Geometry: final body of the model. Coordinates: model frame, mm. Face numbers are marked on the shaded views. A direction names the side the tool comes from. Give positions to 0.01 mm unless a question says otherwise; leave off trailing zeros. Loops run counter-clockwise (first coordinate to the right, second up) from the corner with the lowest first, then second, coordinate; pieces in that order, holes last. Notation, with made-up numbers: (35, 64.25) -> (69, 64.25) arc R16 ccw to (69, 68.25) -> close; hole circle Ø11 at (-27.75, 89.5). An arc over 180 degrees is marked (long way). Answer in a Markdown table with one row per item. Add a question column.
1) Line query: line 1 (X direction, y = 60.5, z = 172); line 2 (X direction, y = 60, z = 145.5); line 3 (Z direction, x = -308.8, y = 196.5). Output: solid intervals per line, ascending. Write a range as from..to.
2) First-contact query: P1, Ø3.5, axis at x = -308.5, y = 141.5, coming from the +Z side; P2, Ø5.5, axis at y = 141, z = 176, coming from the -X side; P3, Ø3.5, axis at y = 207.5, z = 187.5, coming from the +X side. Flat tips, straight axial feed; report the tip coordinate or a pass-through.
3) Access query for the marked faces 1, 2 and 3. Directions: +Z, -Z, +X, -X, +Y, -Y. A direction counts if a zero-diameter tool reaches every point of the face in a straight line with its end or side. Return the directions, or none.
4) Draft query along X for the marked faces 4, 5 and 6. Return one class per face: +X half, -X half, draft (parallel to the pull), parting line (faces both ways), or undercut.
5) Section query C-C (x = -108). Return the cut outline in (y, z), plus the area to 3 significant figures.
6) Section query A-A (y = 176). Return the cut outline in (x, z), plus the area to 3 significant figures.
7) Section query B-B (z = 85.5). Return the cut outline in (x, y).
```python
from build123d import *

# Parameters (mm, degrees)
BASE_FLANGE1_DEPTH             = 186
EDGE_FLANGE1_DEPTH             = 613
M6_CLEARANCE_HOLE1_D           = 6.4
EDGE_FLANGE2_STRIP_W           = 10
EDGE_FLANGE2_STRIP_H           = 1.5
EDGE_FLANGE2_STRIP_CUT_DEPTH   = 186.5
EDGE_FLANGE2_STRIP_2_W         = 10
EDGE_FLANGE2_STRIP_2_H         = 1.5
EDGE_FLANGE2_STRIP_CUT_2_DEPTH = 186.5
EDGE_FLANGE2_DEPTH             = 186.5
EDGE_FLANGE2_BEND_DEPTH        = 186.5
SKETCH17_R                     = 2.05
CUT_EXTRUDE1_DEPTH             = 681.27365817
LPATTERN1_COUNT                = 4
LPATTERN1_PITCH                = 55.5
FILLET1_R                      = 22
FILLET2_R                      = 5
M8_CLEARANCE_HOLE1_D           = 8.4


# Sheet-metal steps are written as plain solids
with BuildPart() as part:
    # Sketch1 → Base-Flange1 (new body)
    with BuildSketch(Plane.XY):
        with BuildLine():
            Line((-308, 0), (-308, 206.5))
            ThreePointArc((-308, 206.5), (-307.560660172, 207.560660172), (-306.5, 208))
            Line((-306.5, 208), (306.5, 208))
            ThreePointArc((306.5, 208), (307.560660172, 207.560660172), (308, 206.5))
            Line((308, 206.5), (308, 0))
            Line((308, 0), (309.5, 0))
            Line((309.5, 0), (309.5, 206.5))
            ThreePointArc((309.5, 206.5), (308.621320344, 208.621320344), (306.5, 209.5))
            Line((306.5, 209.5), (-306.5, 209.5))
            ThreePointArc((-306.5, 209.5), (-308.621320344, 208.621320344), (-309.5, 206.5))
            Line((-309.5, 206.5), (-309.5, 0))
            Line((-309.5, 0), (-308, 0))
        make_face()
    extrude(amount=BASE_FLANGE1_DEPTH)

    # Edge-Flange1 section (across the edge) → Edge-Flange1 (add)
    with BuildSketch(Plane(origin=(306.5, 208, 187.5), x_dir=(0, 0, -1), z_dir=(-1, 0, 0))):
        with BuildLine():
            Line((-1.5, 1.5), (-1.5, 188))
            Line((-1.5, 188), (0, 188))
            Line((0, 188), (0, 1.5))
            ThreePointArc((0, 1.5), (0.439339828, 0.439339828), (1.5, 0))
            Line((1.5, 0), (1.5, -1.5))
            ThreePointArc((1.5, -1.5), (-0.621320344, -0.621320344), (-1.5, 1.5))
        make_face()
    extrude(amount=EDGE_FLANGE1_DEPTH)

    # M6 Clearance Hole1 (through all)
    with Locations(Plane(origin=(0, 209.5, 0), x_dir=(1, 0, 0), z_dir=(0, 1, 0))):
        with Locations((-199.845948124, -14), (-169.845948124, -14)):
            m6_clearance_hole1 = Hole(M6_CLEARANCE_HOLE1_D / 2)

    # Mirror1: M6 Clearance Hole1 across plane
    add(m6_clearance_hole1.mirror(Plane(origin=(0, 0, 0), x_dir=(0, 0, 1), z_dir=(1, 0, 0))), mode=Mode.SUBTRACT)

    # Edge-Flange2 strip (across the edge) → Edge-Flange2 strip cut (cut)
    with BuildSketch(Plane(origin=(-307.5, 20, 187.5), x_dir=(1, 0, 0), z_dir=(0, 1, 0))):
        with Locations((-2, -0.75)):
            Rectangle(EDGE_FLANGE2_STRIP_W, EDGE_FLANGE2_STRIP_H)
    extrude(amount=EDGE_FLANGE2_STRIP_CUT_DEPTH, mode=Mode.SUBTRACT)

    # Edge-Flange2 strip 2 (across the edge) → Edge-Flange2 strip cut 2 (cut)
    with BuildSketch(Plane(origin=(307.5, 206.5, 187.5), x_dir=(-1, 0, 0), z_dir=(0, -1, 0))):
        with Locations((-2, -0.75)):
            Rectangle(EDGE_FLANGE2_STRIP_2_W, EDGE_FLANGE2_STRIP_2_H)
    extrude(amount=EDGE_FLANGE2_STRIP_CUT_2_DEPTH, mode=Mode.SUBTRACT)

    # Edge-Flange2 section (across the edge) → Edge-Flange2 (add)
    with BuildSketch(Plane(origin=(-307.5, 20, 187.5), x_dir=(1, 0, 0), z_dir=(0, 1, 0))):
        with BuildLine():
            Line((0, 1.5), (0, 18.5))
            Line((0, 18.5), (1.5, 18.5))
            Line((1.5, 18.5), (1.5, 1.5))
            ThreePointArc((1.5, 1.5), (1.939339828, 0.439339828), (3, 0))
            Line((3, 0), (3, -1.5))
            ThreePointArc((3, -1.5), (0.878679656, -0.621320344), (0, 1.5))
        make_face()
    extrude(amount=EDGE_FLANGE2_DEPTH)

    # Edge-Flange2 section 2 (across the edge) → Edge-Flange2 bend (add)
    with BuildSketch(Plane(origin=(307.5, 206.5, 187.5), x_dir=(-1, 0, 0), z_dir=(0, -1, 0))):
        with BuildLine():
            Line((0, 1.5), (0, 18.5))
            Line((0, 18.5), (1.5, 18.5))
            Line((1.5, 18.5), (1.5, 1.5))
            ThreePointArc((1.5, 1.5), (1.939339828, 0.439339828), (3, 0))
            Line((3, 0), (3, -1.5))
            ThreePointArc((3, -1.5), (0.878679656, -0.621320344), (0, 1.5))
        make_face()
    extrude(amount=EDGE_FLANGE2_BEND_DEPTH)

    # Sketch17 → Cut-Extrude1 (cut, through all)
    with BuildSketch(Plane.ZY.offset(309.5)):
        with Locations((176, 196.5)):
            Circle(SKETCH17_R)
    cut_extrude1 = extrude(amount=-CUT_EXTRUDE1_DEPTH, mode=Mode.SUBTRACT)

    # LPattern1: Cut-Extrude1 ×4
    with Locations(*[(0, -i * LPATTERN1_PITCH, 0) for i in range(1, LPATTERN1_COUNT)]):
        add(cut_extrude1, mode=Mode.SUBTRACT)

    # Fillet1
    fillet1_edges = [part.edges().sort_by_distance(p)[0] for p in [
        (-308.75, 0, 186),
        (308.75, 0, 186),
    ]]
    fillet(fillet1_edges, radius=FILLET1_R)

    # Fillet2
    fillet2_edges = [part.edges().sort_by_distance(p)[0] for p in [
        (-308.75, 0, 0),
        (-306.75, 20, 169),
        (-306.75, 206.5, 169),
        (308.75, 0, 0),
        (306.75, 206.5, 169),
        (306.75, 20, 169),
    ]]
    fillet(fillet2_edges, radius=FILLET2_R)

    # M8 Clearance Hole1 (through all)
    with Locations(Plane.XY.offset(189)):
        with Locations((-66, 50), (66, 50)):
            Hole(M8_CLEARANCE_HOLE1_D / 2)


solid = part.part
```
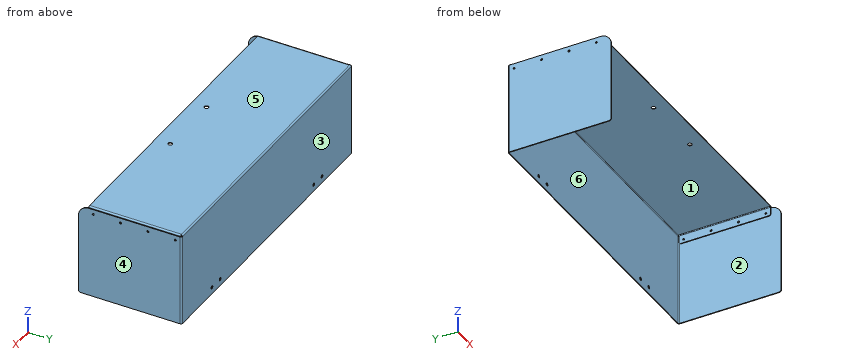
Evaluation:
| question | item | result |
|---|---|---|
| 1 | line 1 | -309.5..-308, -307.5..-306, 306..307.5, 308..309.5 |
| 1 | line 2 | -309.5..-308, 308..309.5 |
| 1 | line 3 | 0..173.95, 178.05..186 |
| 2 | P1 | z = 187.98 |
| 2 | P2 | x = -309.5 |
| 2 | P3 | x = 309.5 |
| 3 | face 1 | -Z, -Y |
| 3 | face 2 | +Z, -Z, -Y |
| 3 | face 3 | +Z, -Z, +X, -X, +Y |
| 4 | face 4 | +X half |
| 4 | face 5 | draft |
| 4 | face 6 | undercut |
| 5 | outline | (20, 187.5) -> (206.5, 187.5) arc R1.5 cw to (208, 186) -> (208, 0) -> (209.5, 0) -> (209.5, 186) arc R3 ccw to (206.5, 189) -> (20, 189) -> close |
| 5 | area | 564 mm² |
| 6 | outline | (-309.5, 0) -> (-308, 0) -> (-308, 186) -> (-309.5, 186) -> close; (-307.5, 169) -> (-306, 169) -> (-306, 186) arc R1.5 cw to (-304.5, 187.5) -> (304.5, 187.5) arc R1.5 cw to (306, 186) -> (306, 169) -> (307.5, 169) -> (307.5, 186) arc R3 ccw to (304.5, 189) -> (-304.5, 189) arc R3 ccw to (-307.5, 186) -> close; (308, 0) -> (309.5, 0) -> (309.5, 186) -> (308, 186) -> close |
| 6 | area | 1,530 mm² |
| 7 | outline | (-309.5, 0) -> (-308, 0) -> (-308, 206.5) arc R1.5 cw to (-306.5, 208) -> (306.5, 208) arc R1.5 cw to (308, 206.5) -> (308, 0) -> (309.5, 0) -> (309.5, 206.5) arc R3 ccw to (306.5, 209.5) -> (-306.5, 209.5) arc R3 ccw to (-309.5, 206.5) -> close |
